Source: three-view drawing plus pictorial views. Frame: mm from the lowest corner of the part. Coordinates: 2 decimals unless noted, no trailing zeros. Order: outer loops, then holes, each group sorted by start corner. A loop starts at its lowest first (then second) coordinate and runs counter-clockwise, first axis right, second up. Notation, with made-up numbers: (15.25, 75.25) -> (60.25, 75.25) arc R28 ccw to (60.25, 95.25) -> close; hole circle Ø3 at (40.25, 25). An arc over 180 degrees is marked (long way). Use one line per item in the form item = value. Start each with the question number.
1) Pin query (flat end, axial travel): pin 1 (4 mm diameter, centred on x = 30, z = 10.5, fed in from -Y). Return the tip coordinate at first contact, or that it passes through.
2) Section query C-C on x = 45. Output: boundary loops of the cut face in (y, z) (3 decimals), then the cut area to 3 significant figures.
3) Section query A-A on z = 10.5. Output: boundary loops of the cut face in (x, y) (3 decimals), then the cut area to 3 significant figures.
4) Section query B-B on x = 74.5. Output: boundary loops of the cut face in (y, z) (3 decimals), then the cut area to 3 significant figures.
5) Section query D-D on y = 1.25. Count the separate pieces of the cut face and the enclosed holes in it, then the cut area to 3 significant figures.
6) Ray query, line 1 along X through (y, z) = (4, 57.5); line 2 along Z through (x, y) = (10, 3.25); line 3 along X through (y, z) = (2, 4.5). Return the intervals inside material, ascending.
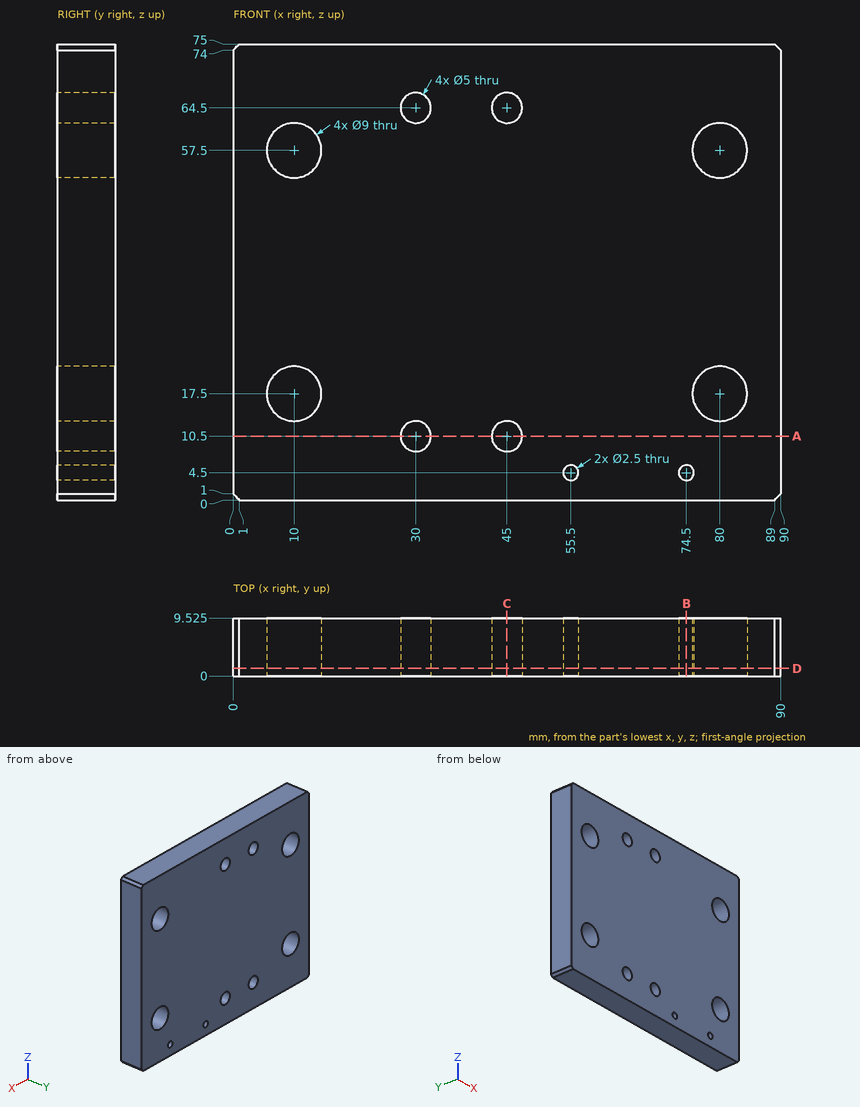
Answers below:
q1.pin_1 = through
q2.outline = (0, 0) -> (9.525, 0) -> (9.525, 8) -> (0, 8) -> close; (0, 13) -> (9.525, 13) -> (9.525, 62) -> (0, 62) -> close; (0, 67) -> (9.525, 67) -> (9.525, 75) -> (0, 75) -> close
q2.area = 619 mm^2
q3.outline = (0, 0) -> (27.5, 0) -> (27.5, 9.525) -> (0, 9.525) -> close; (32.5, 0) -> (42.5, 0) -> (42.5, 9.525) -> (32.5, 9.525) -> close; (47.5, 0) -> (90, 0) -> (90, 9.525) -> (47.5, 9.525) -> close
q3.area = 762 mm^2
q4.outline = (0, 0) -> (9.525, 0) -> (9.525, 3.25) -> (0, 3.25) -> close; (0, 5.75) -> (9.525, 5.75) -> (9.525, 75) -> (0, 75) -> close
q4.area = 691 mm^2
q5.separate_pieces = 1
q5.enclosed_holes = 10
q5.area = 6,410 mm^2
q6.line_1 = 0 to 5.5, 14.5 to 75.5, 84.5 to 90
q6.line_2 = 0 to 13, 22 to 53, 62 to 75
q6.line_3 = 0 to 54.25, 56.75 to 73.25, 75.75 to 90
